```python
from build123d import *

# Parameters (mm, degrees)
SKETCH1_R           = 4
BOSS_EXTRUDE1_DEPTH = 15
SKETCH2_W           = 70
SKETCH2_H           = 60
SKETCH2_R           = 26
SKETCH2_R_2         = 3
BOSS_EXTRUDE3_DEPTH = 67


with BuildPart() as part:
    # Sketch1 → Boss-Extrude1 (new body)
    # profile 1 of 3: a face of its own
    with BuildSketch(Plane(origin=(0, 0, 0), x_dir=(1, 0, 0), z_dir=(0, 1, 0))):
        Polygon((37, 33.5), (-37, 33.5), (-113, 33.5), (-113, -33.5), (-37, -33.5), (37, -33.5), (113, -33.5), (113, 33.5), align=None)
        with Locations(Location((-102, -25, 0), (0, 0, 270))):
            Circle(SKETCH1_R, mode=Mode.SUBTRACT)
        with Locations(Location((-48, -25, 0), (0, 0, 270))):
            Circle(SKETCH1_R, mode=Mode.SUBTRACT)
        with Locations(Location((48, -25, 0), (0, 0, 270))):
            Circle(SKETCH1_R, mode=Mode.SUBTRACT)
        with Locations(Location((102, -25, 0), (0, 0, 270))):
            Circle(SKETCH1_R, mode=Mode.SUBTRACT)
        with Locations(Location((-102, 25, 0), (0, 0, 270))):
            Circle(SKETCH1_R, mode=Mode.SUBTRACT)
        with Locations(Location((-48, 25, 0), (0, 0, 270))):
            Circle(SKETCH1_R, mode=Mode.SUBTRACT)
        with Locations(Location((48, 25, 0), (0, 0, 270))):
            Circle(SKETCH1_R, mode=Mode.SUBTRACT)
        with Locations(Location((102, 25, 0), (0, 0, 270))):
            Circle(SKETCH1_R, mode=Mode.SUBTRACT)
    # profile 2 of 3: a face of its own
    with BuildSketch(Plane(origin=(0, 0, 0), x_dir=(1, 0, 0), z_dir=(0, 1, 0))):
        Polygon((37, 33.5), (-37, 33.5), (-113, 33.5), (-113, -33.5), (-37, -33.5), (37, -33.5), (113, -33.5), (113, 33.5), align=None)
        with Locations(Location((-102, -25, 0), (0, 0, 270))):
            Circle(SKETCH1_R, mode=Mode.SUBTRACT)
        with Locations(Location((-48, -25, 0), (0, 0, 270))):
            Circle(SKETCH1_R, mode=Mode.SUBTRACT)
        with Locations(Location((48, -25, 0), (0, 0, 270))):
            Circle(SKETCH1_R, mode=Mode.SUBTRACT)
        with Locations(Location((102, -25, 0), (0, 0, 270))):
            Circle(SKETCH1_R, mode=Mode.SUBTRACT)
        with Locations(Location((-102, 25, 0), (0, 0, 270))):
            Circle(SKETCH1_R, mode=Mode.SUBTRACT)
        with Locations(Location((-48, 25, 0), (0, 0, 270))):
            Circle(SKETCH1_R, mode=Mode.SUBTRACT)
        with Locations(Location((48, 25, 0), (0, 0, 270))):
            Circle(SKETCH1_R, mode=Mode.SUBTRACT)
        with Locations(Location((102, 25, 0), (0, 0, 270))):
            Circle(SKETCH1_R, mode=Mode.SUBTRACT)
    # profile 3 of 3: a face of its own
    with BuildSketch(Plane(origin=(0, 0, 0), x_dir=(1, 0, 0), z_dir=(0, 1, 0))):
        Polygon((37, 33.5), (-37, 33.5), (-113, 33.5), (-113, -33.5), (-37, -33.5), (37, -33.5), (113, -33.5), (113, 33.5), align=None)
        with Locations(Location((-102, -25, 0), (0, 0, 270))):
            Circle(SKETCH1_R, mode=Mode.SUBTRACT)
        with Locations(Location((-48, -25, 0), (0, 0, 270))):
            Circle(SKETCH1_R, mode=Mode.SUBTRACT)
        with Locations(Location((48, -25, 0), (0, 0, 270))):
            Circle(SKETCH1_R, mode=Mode.SUBTRACT)
        with Locations(Location((102, -25, 0), (0, 0, 270))):
            Circle(SKETCH1_R, mode=Mode.SUBTRACT)
        with Locations(Location((-102, 25, 0), (0, 0, 270))):
            Circle(SKETCH1_R, mode=Mode.SUBTRACT)
        with Locations(Location((-48, 25, 0), (0, 0, 270))):
            Circle(SKETCH1_R, mode=Mode.SUBTRACT)
        with Locations(Location((48, 25, 0), (0, 0, 270))):
            Circle(SKETCH1_R, mode=Mode.SUBTRACT)
        with Locations(Location((102, 25, 0), (0, 0, 270))):
            Circle(SKETCH1_R, mode=Mode.SUBTRACT)
    extrude(amount=BOSS_EXTRUDE1_DEPTH)

    # Sketch2 → Boss-Extrude3 (add)
    with BuildSketch(Plane.XY.offset(33.5)):
        with Locations((0, -25.75)):
            Rectangle(SKETCH2_W, SKETCH2_H)
        with Locations((0, -25.75)):
            Circle(SKETCH2_R, mode=Mode.SUBTRACT)
        with Locations((-29.011851027, -9)):
            Circle(SKETCH2_R_2, mode=Mode.SUBTRACT)
        with Locations((-29.011851027, -42.5)):
            Circle(SKETCH2_R_2, mode=Mode.SUBTRACT)
        with Locations((29.011851027, -42.5)):
            Circle(SKETCH2_R_2, mode=Mode.SUBTRACT)
        with Locations((29.011851027, -9)):
            Circle(SKETCH2_R_2, mode=Mode.SUBTRACT)
    extrude(amount=-BOSS_EXTRUDE3_DEPTH)


solid = part.part
```
Can you work these out from the model? Positions are in its coordinate system, mm. A direction names the side the tool comes from. Give positions to 0.01 mm unless a question says otherwise; leave off trailing zeros. Write each loop counter-clockwise with the first axis right and the second up, starting at its lowest first coordinate (ties: lowest second). Pieces come first, ordered by that corner, then holes. Notation, with made-up numbers: (60.25, 58) -> (110.25, 58) arc R10 ccw to (110.25, 77) -> close; hole circle Ø9 at (29.25, -34). An arc over 180 degrees is marked (long way). Write item = value, one per line.
(1) For faces 4 (the face through (98.095, 7.395, -25.867)), 5 (the face through (0, 0, 0)), 6 (the face through (-35, -28, 0)), 7 (the face through (35, -28, 0)), which set-ups out of +Z, -Z, +X, -X, +Y, -Y let a thin tool reach every point of the face, with its end or its side?
Worked out:
face_4 = +Y, -Y
face_5 = +Z, -Z
face_6 = +Z, -Z, -X, -Y
face_7 = +Z, -Z, +X, -Y
(2) Thinking about a two-plate mould opening in Y: for faces 1 (the face through (-1, 3, -33.5)), 2 (the face through (-31.22, -40.47, 0.47)), 3 (the face through (73, 0, 0)), which applies, released by +Y, released by -Y, zero draft, split by the parting line, or undercut?
Worked out:
face_1 = zero draft
face_2 = undercut
face_3 = released by -Y
(3) I'm going to push flat-ended pins straight in: P1, Ø5.5, axis at x = 29.01, y = -42.5, coming from the -Z side; P2, Ø10, axis at y = -43.5, z = -22.5, coming from the +X side; P3, Ø12, axis at y = -26, z = -18, coming from the -X side. Where does each tip first touch, or does it pass through?
Worked out:
P1 = through
P2 = 35
P3 = -35
(4) Suppose I cut it at B-B on z = -25. Count the separate pieces of the cut face and the enclosed holes in it, then the cut area to 3 significant figures.
Worked out:
separate_pieces = 5
enclosed_holes = 5
area = 4,580 mm^2
(5) I need wall thicknesses on probe 1 along X at (y, z) = (8, -25); probe 2 along Y at (x, z) = (0, -11); probe 3 along X at (y, z) = (-26, -11). Which ranges of each line are inside material? Lowest first, please. Write a range as from..to.
Worked out:
probe_1 = -113..-106, -98..-52, -44..44, 52..98, 106..113
probe_2 = -55.75..-51.75, 0..15
probe_3 = -35..-26, 26..35
(6) Suppose I cut it at D-D on y = -30.5. Write out the boundary of the cut face in (x, z).
Worked out:
outline = (-35, -33.5) -> (-25.56, -33.5) -> (-25.56, 33.5) -> (-35, 33.5) -> close; (25.56, -33.5) -> (35, -33.5) -> (35, 33.5) -> (25.56, 33.5) -> close
(7) Suppose I cut it at A-A on x = 0. Write out the boundary of the cut face in (y, z), then the cut area to 3 significant figures.
Worked out:
outline = (-55.75, -33.5) -> (-51.75, -33.5) -> (-51.75, 33.5) -> (-55.75, 33.5) -> close; (0, -33.5) -> (15, -33.5) -> (15, 33.5) -> (0, 33.5) -> close
area = 1,270 mm^2
(8) Suppose I cut it at C-C on z = -1. Write out the boundary of the cut face in (x, y), then the cut area to 3 significant figures.
Worked out:
outline = (-113, 0) -> (-35, 0) -> (-35, -55.75) -> (35, -55.75) -> (35, 0) -> (113, 0) -> (113, 15) -> (-113, 15) -> close; hole circle Ø6 at (-29.01, -42.5); hole circle Ø6 at (-29.01, -9); hole (-3.6, 0) arc R26 ccw (long way) to (3.6, 0) -> close; hole circle Ø6 at (29.01, -42.5); hole circle Ø6 at (29.01, -9)
area = 5,060 mm^2
